Read the model definition and answer for the solid it produces. Units are mm, in the model's axes. Coordinates: 2 decimals unless noted, no trailing zeros. Write each loop counter-clockwise with the first axis right and the second up, starting at its lowest first coordinate (ties: lowest second). Pieces come first, ordered by that corner, then holes.
(1) The part is cut by section A-A, the plane x = 52. Determine the outline of the cut face in (y, z) (3 decimals), and give its area (3 significant figures).
(2) The part is cut by section B-B, the plane x = 112.5. Determine the outline of the cut face in (y, z), and give its area (3 significant figures).
(3) Straight lines are drawn through the part: line 1 along Z through (x, y) = (60, 2.05) (3 decimals); line 2 along X through (y, z) = (3.15, -7.5); line 3 along Z through (x, y) = (7.5, 2.05). For each, find the intervals that lie inside material, in ascending order.
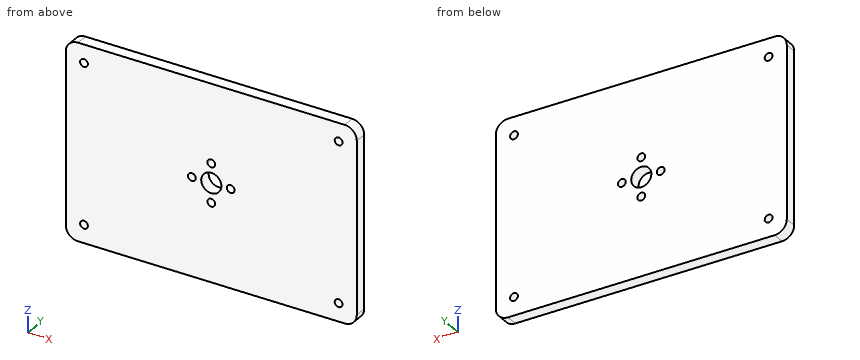
```python
from build123d import *

# Parameters (mm, degrees)
SKETCH1_W           = 120
SKETCH1_H           = 80.79
SKETCH1_R           = 1.6
SKETCH1_R_2         = 4.15
BOSS_EXTRUDE1_DEPTH = 5
SKETCH2_R           = 1.6
CUT_EXTRUDE1_DEPTH  = 6
FILLET1_R           = 5


with BuildPart() as part:
    # Sketch1 → Boss-Extrude1 (new body)
    with BuildSketch(Plane(origin=(0, 0, 0), x_dir=(1, 0, 0), z_dir=(0, 1, 0))):
        with Locations((60, 40.395)):
            Rectangle(SKETCH1_W, SKETCH1_H)
        with Locations((52, 40.395)):
            Circle(SKETCH1_R, mode=Mode.SUBTRACT)
        with Locations((60, 48.395)):
            Circle(SKETCH1_R, mode=Mode.SUBTRACT)
        with Locations((68, 40.395)):
            Circle(SKETCH1_R, mode=Mode.SUBTRACT)
        with Locations((60, 32.395)):
            Circle(SKETCH1_R, mode=Mode.SUBTRACT)
        with Locations((60, 40.395)):
            Circle(SKETCH1_R_2, mode=Mode.SUBTRACT)
    extrude(amount=BOSS_EXTRUDE1_DEPTH)

    # Sketch2 → Cut-Extrude1 (cut, through all)
    with BuildSketch(Plane(origin=(0, 5, 0), x_dir=(1, 0, 0), z_dir=(0, 1, 0))):
        with Locations((7.5, 7.5)):
            Circle(SKETCH2_R)
        with Locations((7.5, 73.29)):
            Circle(SKETCH2_R)
        with Locations((112.5, 7.5)):
            Circle(SKETCH2_R)
        with Locations((112.5, 73.29)):
            Circle(SKETCH2_R)
    extrude(amount=-CUT_EXTRUDE1_DEPTH, mode=Mode.SUBTRACT)

    # Fillet1
    fillet1_edges = [part.edges().sort_by_distance(p)[0] for p in [
        (0, 2.5, -80.79),
        (120, 2.5, -80.79),
        (120, 2.5, 0),
        (0, 2.5, 0),
    ]]
    fillet(fillet1_edges, radius=FILLET1_R)


solid = part.part
```
Computed:
1. outline: (0, -80.79) - (5, -80.79) - (5, -41.995) - (0, -41.995) - close; (0, -38.795) - (5, -38.795) - (5, 0) - (0, 0) - close
1. area: 388 mm2
2. outline: (0, -80.79) - (5, -80.79) - (5, -74.89) - (0, -74.89) - close; (0, -71.69) - (5, -71.69) - (5, -9.1) - (0, -9.1) - close; (0, -5.9) - (5, -5.9) - (5, 0) - (0, 0) - close
2. area: 372 mm2
3. line 1: z = -80.79 to -49.995, -46.795 to -44.545, -36.245 to -33.995, -30.795 to 0
3. line 2: x = 0 to 5.9, 9.1 to 110.9, 114.1 to 120
3. line 3: z = -80.79 to -74.89, -71.69 to -9.1, -5.9 to 0
